from build123d import *

# Parameters (mm, degrees)
F1_DEPTH = 20
F2_DEPTH = 15.2
F4_DEPTH = 15


with BuildPart() as f1:
    # F0 (on Top) → F1 (new body)
    with BuildSketch(Plane.XY):
        Polygon((-40, 0), (0, 0), (0, 20), (-15, 20), (-10, 11.339746), (-32.8, 11.339746), (-27.8, 20), (-40, 20), align=None)
        Polygon((0, 20), (0, 0), (40, 0), (40, 20), (27.8, 20), (32.8, 11.339746), (10, 11.339746), (15, 20), align=None)
        Polygon((-10, 11.339746), (-15, 20), (-27.8, 20), (-32.8, 11.339746), align=None)
        Polygon((27.8, 20), (15, 20), (10, 11.339746), (32.8, 11.339746), align=None)
    extrude(amount=-F1_DEPTH)

    # F0 (on Top) → F2 (cut)
    with BuildSketch(Plane.XY):
        Polygon((-10, 11.339746), (-15, 20), (-27.8, 20), (-32.8, 11.339746), align=None)
        Polygon((27.8, 20), (15, 20), (10, 11.339746), (32.8, 11.339746), align=None)
    extrude(amount=-F2_DEPTH, mode=Mode.SUBTRACT)

    # F3 (on face) → F4 (cut)
    with BuildSketch(Plane.XZ):
        with BuildLine():
            ThreePointArc((4.25, -10), (3.005204, -6.994796), (0, -5.75))
            Line((0, -5.75), (0, -10))
            Line((0, -10), (0, -14.25))
            ThreePointArc((0, -14.25), (3.005204, -13.005204), (4.25, -10))
        make_face()
        with BuildLine():
            Line((0, -10), (0, -5.75))
            ThreePointArc((0, -5.75), (-4.25, -10), (0, -14.25))
            Line((0, -14.25), (0, -10))
        make_face()
    extrude(amount=-F4_DEPTH, mode=Mode.SUBTRACT)


solid = f1.part
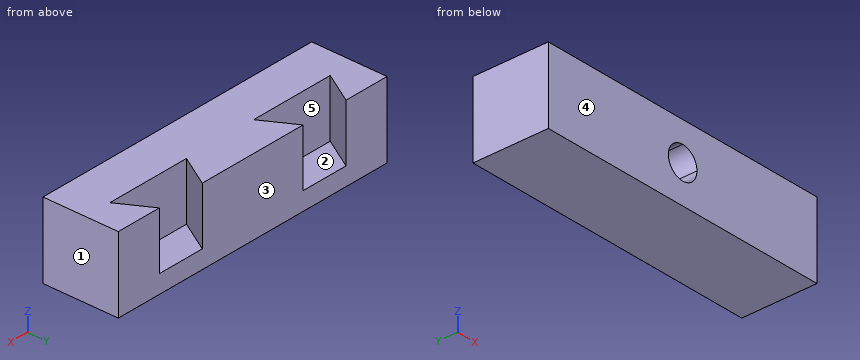
The listing builds one solid part. Answer for the finished solid, in the listing's coordinates (mm). Face numbers are marked on the shaded views. A direction names the side the tool comes from. Give positions to 0.01 mm unless a question says otherwise; leave off trailing zeros. Write each loop counter-clockwise with the first axis right and the second up, starting at its lowest first coordinate (ties: lowest second). Pieces come first, ordered by that corner, then holes.
1) Given P1, Ø2.5, axis at x = 26.5, y = 14, coming from the +Z side; P2, Ø12, axis at x = -21.5, z = -9, coming from the +Y side, each flat-ended and moving along its own axis, determine where each tip first touches the part or whether it passes through.
2) A tool of negligible diameter and unlimited length cuts with its end or side. For the marked faces 1 and 2, from which of +Z, -Z, +X, -X, +Y, -Y can it reach the whole face along a straight path? Write none if from no direction.
3) Section B-B (x = -13) is taken. Write down the section's boundary in (y, z), and give its area (3 significant figures).
4) Section D-D (x = 21.5) is taken. Write down the section's boundary in (y, z), and give its area (3 significant figures).
5) Section A-A (y = 7.5) is taken. Write down the section's boundary in (x, z).
6) For a pull along Y with two mould halves and no side action, classify the marked faces 3, 4 and 5 as pulls with the +Y half, pulls with the -Y half, needs draft (parallel to the pull), parting line crosses it, or undercut.
7) Section C-C (z = -11.5) is taken. Write down the section's boundary in (x, y).
8) Find the intervals of material crossed by L1, parallel to X at y = 12.25, z = -2.5; L2, parallel to X at y = 16.5, z = -10.25; L3, parallel to X at y = 14, z = -10.5, in increasing order.
Response:
1. P1: stops at z = -15.2
1. P2: stops at y = 11.34
2. face 1: +Z, -Z, +X, +Y, -Y
2. face 2: +Z
3. outline: (0, -20) - (20, -20) - (20, 0) - (16.54, 0) - (16.54, -15.2) - (11.34, -15.2) - (11.34, 0) - (0, 0) - close
3. area: 321 mm2
4. outline: (0, -20) - (20, -20) - (20, -15.2) - (11.34, -15.2) - (11.34, 0) - (0, 0) - close
4. area: 268 mm2
5. outline: (-40, -20) - (40, -20) - (40, 0) - (-40, 0) - close; hole circle Ø8.5 at (0, -10)
6. face 3: pulls with the +Y half
6. face 4: pulls with the -Y half
6. face 5: undercut
7. outline: (-40, 0) - (-3.98, 0) - (-3.98, 15) - (3.98, 15) - (3.98, 0) - (40, 0) - (40, 20) - (27.8, 20) - (32.8, 11.34) - (10, 11.34) - (15, 20) - (-15, 20) - (-10, 11.34) - (-32.8, 11.34) - (-27.8, 20) - (-40, 20) - close
8. L1: x = -40 to -32.27, -10.53 to 10.53, 32.27 to 40
8. L2: x = -40 to -29.82, -12.98 to 12.98, 29.82 to 40
8. L3: x = -40 to -31.26, -11.54 to -4.22, 4.22 to 11.54, 31.26 to 40
